Here's the drawing with two shaded views (mm, measured from the low corner). I have some questions. Give positions to 0.01 mm unless a question says otherwise; leave off trailing zeros. Write each loop counter-clockwise with the first axis right and the second up, starting at its lowest first coordinate (ties: lowest second). Pieces come first, ordered by that corner, then holes.
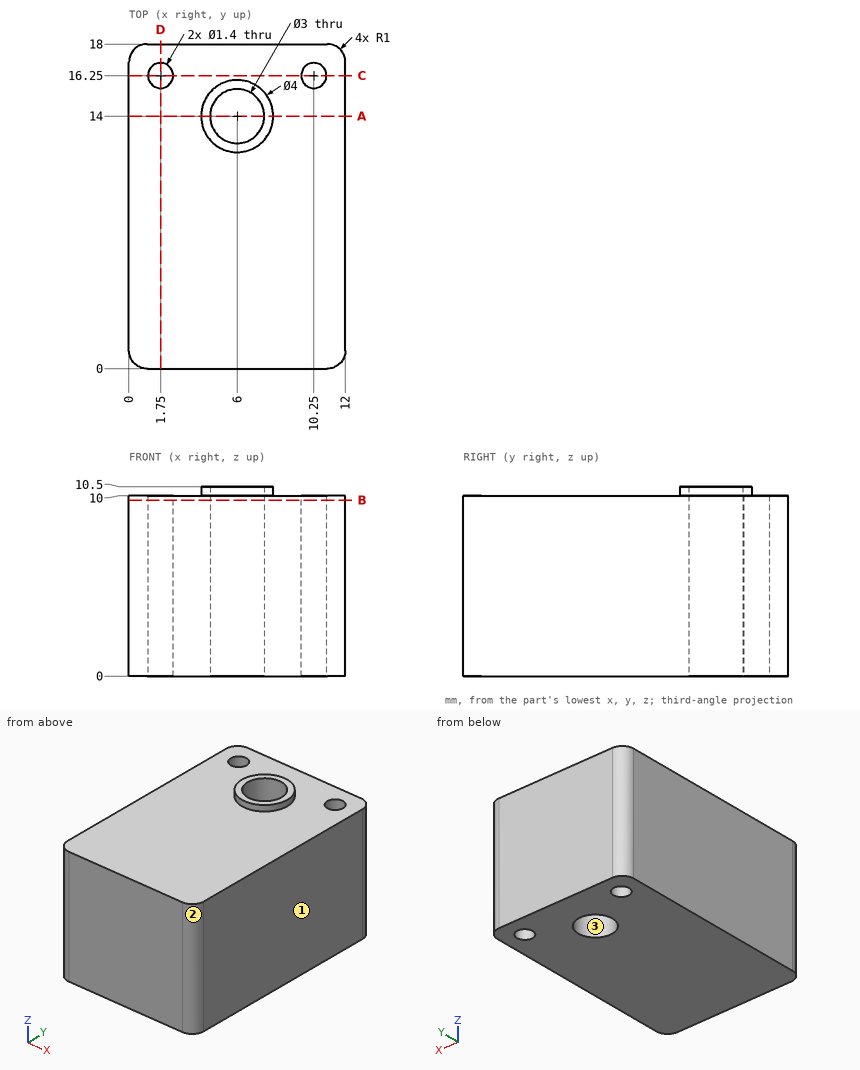
(1) Will these pins go through, and if not, where does the flat tip stop? P1, Ø1.3, axis at x = 10.25, y = 16.25, coming from the +Z side; P2, Ø3.5, axis at x = 8.5, y = 4.5, coming from the +Z side.
Returned:
P1: passes through
P2: stops at z = 10
(2) Imagine slicing it at B-B, the plane z = 9.75. Write out the boundary of the cut face in (x, y), plus the area to 3 significant figures.
Returned:
outline: (0, 1) arc R1 ccw to (1, 0) - (11, 0) arc R1 ccw to (12, 1) - (12, 17) arc R1 ccw to (11, 18) - (1, 18) arc R1 ccw to (0, 17) - close; hole circle Ø1.4 at (1.75, 16.25); hole circle Ø3 at (6, 14); hole circle Ø1.4 at (10.25, 16.25)
area: 205 mm2
(3) If I drill on L1, parallel to X at y = 16.25, z = 8; L2, parallel to Y at x = 1.75, z = 4.25; L3, parallel to Y at x = 6, z = 7.75, over which ranges is the centre line in solid material (lowest first)?
Returned:
L1: x = 0 to 1.05, 2.45 to 9.55, 10.95 to 12
L2: y = 0 to 15.55, 16.95 to 18
L3: y = 0 to 12.5, 15.5 to 18
(4) If we mould it in two halves opening along Y, with no side actions, what happens to the marked faces 1, 2 and 3? For each: +Y half, -Y half, draft (parallel to the pull), parting line (faces both ways), or undercut.
Returned:
face 1: draft
face 2: -Y half
face 3: undercut
(5) Imagine slicing it at D-D, the plane x = 1.75. Write out the boundary of the cut face in (y, z), plus the area to 3 significant figures.
Returned:
outline: (0, 0) - (15.55, 0) - (15.55, 10) - (0, 10) - close; (16.95, 0) - (18, 0) - (18, 10) - (16.95, 10) - close
area: 166 mm2
(6) Imagine slicing it at C-C, the plane y = 16.25. Write out the boundary of the cut face in (x, z), plus the area to 3 significant figures.
Returned:
outline: (0, 0) - (1.05, 0) - (1.05, 10) - (0, 10) - close; (2.45, 0) - (9.55, 0) - (9.55, 10) - (2.45, 10) - close; (10.95, 0) - (12, 0) - (12, 10) - (10.95, 10) - close
area: 92.0 mm2
(7) Imagine slicing it at A-A, the plane y = 14. Write out the boundary of the cut face in (x, z).
Returned:
outline: (0, 0) - (4.5, 0) - (4.5, 10.5) - (4, 10.5) - (4, 10) - (0, 10) - close; (7.5, 0) - (12, 0) - (12, 10) - (8, 10) - (8, 10.5) - (7.5, 10.5) - close
